Autodesk Inventor part; units mm, degrees
ref_plane "Work Plane1" through (15, 0, 0) normal (0, 0, 1) x (1, 0, 0)
ref_plane "YZ Plane" through (0, 0, 0) normal (1, 0, 0) x (0, 1, 0)
ref_plane "XZ Plane" through (0, 0, 0) normal (0, 1, 0) x (-1, 0, 0)
sketch "Sketch1" plane through (0, 0, 0) normal (0, 0, 1) x (1, 0, 0)
  line L0 (-0.8667, 0) -> (41.25, 0)
  line L1 (41.25, 0) -> (41.25, 3)
  line L2 (41.25, 3) -> (30, 3)
  line L3 (30, 3) -> (30, 4)
  line L4 (30, 4) -> (0, 4)
  line L5 (0, 4) -> (0, 6.5)
  line L6 (0, 6.5) -> (-5.5, 6.5)
  line L7 (-5.5, 6.5) -> (-5.5, 2.3094)
  line L8 (-5.5, 2.3094) -> (-2.2, 2.3094)
  line L9 (-2.2, 2.3094) -> (-0.8667, 0)
  line L10 (-10.175, 0) -> (55.275, 0)
  line L11 (0, -0.65) -> (0, 8.45)
  line L12 (0, 3.71) -> (2.5, 3.71)
  line L13 (2.5, 3.71) -> (2.79, 4)
  line L14 (30, 3) -> (30, 2.3865)
  line L15 (30, 2.3865) -> (30.6134, 2.3865)
  line L16 (30.6134, 2.3865) -> (31.676, 3)
  line L17 (0, 3.71) -> (0, 4)
  dimension "d0" = 6
  dimension "d1" = 8
  dimension "d2" = 13
  dimension "d3" = 4.6188
  dimension "d5" = 11.25
  dimension "d6" = 5.5
  dimension "d7" = 3.3
  dimension "d8" = 60
  dimension "d9" = 41.25
  dimension "d18" = 2.5
  dimension "d19" = 45
  dimension "d20" = 7.42
  dimension "d21" = 4.7731
  dimension "d22" = 30
  dimension "d23" = 0.6135
revolve "Body" add sketch "Sketch1" angle 360 about axis through (-0.8667, 0, 0) along (1, 0, 0)
sketch "Sketch2" plane through (-5.5, 0, 0) normal (-1, 0, 0) x (0, 0, 1)
  circle A0 centre (0, 0) radius 2.3094
  line L0 (0, 2.3094) -> (2, 1.1547)
  line L1 (2, 1.1547) -> (2, -1.1547)
  line L2 (2, -1.1547) -> (0, -2.3094)
  line L3 (0, -2.3094) -> (-2, -1.1547)
  line L4 (-2, -1.1547) -> (-2, 1.1547)
  line L5 (-2, 1.1547) -> (0, 2.3094)
  point P0 (0, 0)
extrude "Slot" add sketch "Sketch2" against normal up to next contours A0 L1 | L0 A0 | A0 L2 | L5 A0 | A0 L3 | L4 A0
fillet "Fillet1" radius 2.3622 1 edges at (-5.5, -6.5, 0)
thread "Thread"
chamfer "Chamfer1" distance 0.6135 distance2 0.6135 1 edges at (41.25, -3, 0) measured on face at (41.25, 1, 0)
chamfer "Chamfer2" distance 1 angle 1 1 edges at (30, -4, 0) measured on face at (30, 3.5989, -0.5584)
revolve "Groove1" cut sketch "Sketch1" angle 360 about axis through (-0.8667, 0, 0) along (1, 0, 0) contours L11 L4 L13 L12
revolve "Groove2" cut sketch "Sketch1" angle 360 about axis through (-0.8667, 0, 0) along (1, 0, 0) contours L16 L15 L14 L2
ref_plane "Work Plane1" through (15, 0, 0) normal (0, 0, 1) x (1, 0, 0)
equation "\"d0\" = NND"
equation "\"d1\" = BDM"
equation "\"d2\" = KOD"
equation "\"d3\" = 1.1547 * SW"
equation "\"d5\" = GEL"
equation "\"d6\" = KOH"
equation "\"d7\" = INTI + LOTI"
equation "\"d8\" = 0.5 * ANG"
equation "\"d9\" = NLG"
equation "\"d18\" = GAL2"
equation "\"d19\" = FAWI4"
equation "\"d20\" = BDMM"
equation "\"d21\" = GD1"
equation "\"d22\" = FAWI2"
equation "\"d23\" = GAL"
equation "\"d13\" = RR"
equation "\"d25\" = GEL"
equation "\"d14\" = -0.5 * SPD + 0.5 * NND"
equation "\"d15\" = GUL"
equation "\"d16\" = -0.5 * NND + 0.5 * BDM"
equation "\"d32\" = -0.5 * NND + 0.5 * BDM"
equation "\"NND\" = 6"
equation "\"NLG\" = 41.25"
equation "\"GEL\" = 11.25"
equation "\"KOD\" = 13"
equation "\"KOH\" = 5.5"
equation "\"INTI\" = 3.3"
equation "\"GAL\" = 0.61345 * PTC"
equation "\"GUL\" = 0.61345 * PTC"
equation "\"SPD\" = NND - 1.2269 * PTC"
equation "\"BDM\" = 8"
equation "\"ANG\" = 120deg"
equation "\"FAWI2\" = 30deg"
equation "\"FAWI3\" = 89deg"
equation "\"FAWI4\" = 45deg"
equation "\"RR\" = 2.3622"
equation "\"SW\" = 4"
equation "\"BDMM\" = 7.42"
equation "\"GAL2\" = 2.5"
equation "\"LOTI\" = 0"
equation "\"GD1\" = THREADDIA - 1.2269 * PTC"
equation "\"PTC\" = 1"
equation "\"BOR\" = 4"
equation "\"THREADDIA\" = 6"
equation "\"E0\" = 1.155 * SW"
equation "\"TOA\" = 30deg"
equation "\"PHH\" = 0.55"
properties part number "100005" material "Steel, Mild"
Source: CAD feature listing. Evaluate the final solid. Frame: model axes, mm. A direction names the side the tool comes from. Round coordinates to 2 decimals unless told otherwise and drop trailing zeros. Loops run counter-clockwise (first coordinate to the right, second up) from the corner with the lowest first, then second, coordinate; pieces in that order, holes last.
Q1. First-contact query: P1, Ø4, axis at x = 10, z = -1, coming from the +Y side; P2, Ø2, axis at x = 5.5, z = 1, coming from the -Y side; P3, Ø3, axis at x = 18, z = -3.5, coming from the +Y side. Flat tips, straight axial feed; report the tip coordinate or a pass-through.
Q2. Ray query, line 1 (X direction, y = -2, z = 1.5); line 2 (Y direction, x = 13, z = -1.5); line 3 (Y direction, x = 2, z = 1). Return the intervals inside material, ascending.
Q3. Access query for faces 4 (the face through (41.25, 0, 0)), 5 (the face through (36, -3, 0)), 6 (the face through (-4, 0, 2)). Directions: +Z, -Z, +X, -X, +Y, -Y. A direction counts if a zero-diameter tool reaches every point of the face in a straight line with its end or side. Return the directions, or none.
Q4. Section B-B, the plane x = 36. Return loops of the section in (y, z).
Q5. Mould query, pull axis X, two halves, no side actions, for faces 1 (the face through (16.196, -0.867, 3.905)), 2 (the face through (-5.5, -2, -1)), 3 (the face through (1.268, -0.804, -3.622)). Classes: pulls with the +X half, pulls with the -X half, needs draft (parallel to the pull), parting line crosses it, or undercut.
Q6. Section A-A, the plane x = 17.5. Return loops of the section in (y, z).
Solutions:
1. P1: stops at y = 4
1. P2: stops at y = -4
1. P3: stops at y = 3.46
2. line 1: x = -5.5 to 30, 30.81 to 41.14
2. line 2: y = -3.71 to 3.71
2. line 3: y = -3.57 to 3.57
3. face 4: +Z, -Z, +X, +Y, -Y
3. face 5: +X
3. face 6: -X
4. outline: circle Ø6 at (0, 0)
5. face 1: needs draft
5. face 2: pulls with the -X half
5. face 3: undercut
6. outline: circle Ø8 at (0, 0)
